Build history of the part. All positions in model axes, mm. Face numbers are marked on the shaded views. Give positions to 0.01 mm unless a question says otherwise; leave off trailing zeros. Loops run counter-clockwise (first coordinate to the right, second up) from the corner with the lowest first, then second, coordinate; pieces in that order, holes last. Notation, with made-up numbers: M -10.75,88 L 19.25,88 A29 cw 19.25,111 Z; hole C 85,-22 d10. An arc over 180 degrees is marked long. Answer in a Markdown table with one row per item. Add a question column.
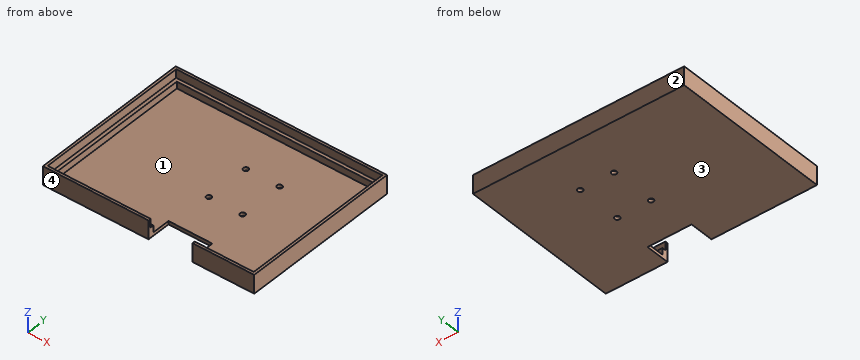
```python
from build123d import *

# Parameters (mm, degrees)
SKETCH1_W           = 125
SKETCH1_H           = 95
SKETCH1_W_2         = 118
SKETCH1_H_2         = 88
BOSS_EXTRUDE1_DEPTH = 4
SKETCH2_W           = 125
SKETCH2_H           = 95
BOSS_EXTRUDE2_DEPTH = 2
SKETCH3_W           = 125
SKETCH3_H           = 95
SKETCH3_W_2         = 122
SKETCH3_H_2         = 92
BOSS_EXTRUDE3_DEPTH = 5
SKETCH5_R           = 1.5
CUT_EXTRUDE1_DEPTH  = 26.5
SKETCH7_W           = 26
SKETCH7_H           = 14.212575567
CUT_EXTRUDE2_DEPTH  = 26.5


with BuildPart() as part:
    # Sketch1 → Boss-Extrude1 (new body)
    with BuildSketch(Plane.XY):
        Rectangle(SKETCH1_W, SKETCH1_H)
        Rectangle(SKETCH1_W_2, SKETCH1_H_2, mode=Mode.SUBTRACT)
    extrude(amount=BOSS_EXTRUDE1_DEPTH)

    # Sketch2 → Boss-Extrude2 (add)
    with BuildSketch(Plane(origin=(0, 0, 0), x_dir=(-1, 0, 0), z_dir=(0, 0, -1))):
        Rectangle(SKETCH2_W, SKETCH2_H)
    extrude(amount=BOSS_EXTRUDE2_DEPTH)

    # Sketch3 → Boss-Extrude3 (add)
    with BuildSketch(Plane.XY.offset(4)):
        Rectangle(SKETCH3_W, SKETCH3_H)
        Rectangle(SKETCH3_W_2, SKETCH3_H_2, mode=Mode.SUBTRACT)
    extrude(amount=BOSS_EXTRUDE3_DEPTH)

    # Sketch5 → Cut-Extrude1 (cut)
    with BuildSketch(Plane(origin=(0, 0, -2), x_dir=(-1, 0, 0), z_dir=(0, 0, -1))):
        with Locations((-23, 18.5)):
            Circle(SKETCH5_R)
        with Locations((-23, -8)):
            Circle(SKETCH5_R)
        with Locations((-3, -8)):
            Circle(SKETCH5_R)
        with Locations((-3, 18.5)):
            Circle(SKETCH5_R)
    extrude(amount=-CUT_EXTRUDE1_DEPTH, mode=Mode.SUBTRACT)

    # Sketch7 → Cut-Extrude2 (cut)
    with BuildSketch(Plane(origin=(0, 0, -2), x_dir=(-1, 0, 0), z_dir=(0, 0, -1))):
        with Locations((-13, -40.393712217)):
            Rectangle(SKETCH7_W, SKETCH7_H)
    extrude(amount=-CUT_EXTRUDE2_DEPTH, mode=Mode.SUBTRACT)


solid = part.part
```
(1) Slice it at D-D, the plane x = 48. Give the cut face in (y, z).
(2) Pin check, flat tips, straight feed: pin 1 (2.5 mm diameter, centred on x = 3, y = 18.5, fed in from -Z); pin 2 (2 mm diameter, centred on x = 16.5, z = -1, fed in from -Y); pin 3 (12 mm diameter, centred on x = -1, y = -3.5, fed in from +Z). Stop position of each tip, or through.
(3) Slice it at B-B, the plane x = 23. Give the cut face in (y, z), then the cut area to 3 significant figures.
(4) Pull direction Y, two halves, no side cores. Call the marked faces 1, 2, 3 and 4: +Y half, -Y half, draft (parallel to the pull), parting line (faces both ways), or undercut.
(5) Slice it at C-C, the plane z = 7. Give the cut face in (x, y).
(6) Wall check: line 1 (Y direction, x = 3, z = -0.75); line 2 (Y direction, x = -3.5, z = 5.5); line 3 (X direction, y = -39, z = 7). Give the ranges that are in metal, low to high.
(7) Slice it at A-A, the plane y = -8. Give the cut face in (x, z).
Solution:
| question | item | result |
|---|---|---|
| 1 | outline | M -47.5,-2 L 47.5,-2 L 47.5,9 L 46,9 L 46,4 L 44,4 L 44,0 L -44,0 L -44,4 L -46,4 L -46,9 L -47.5,9 Z |
| 2 | pin 1 | through |
| 2 | pin 2 | y = -33.29 |
| 2 | pin 3 | z = 0 |
| 3 | outline | M -33.29,-2 L -9.5,-2 L -9.5,0 L -33.29,0 Z; M -6.5,-2 L 17,-2 L 17,0 L -6.5,0 Z; M 20,-2 L 47.5,-2 L 47.5,9 L 46,9 L 46,4 L 44,4 L 44,0 L 20,0 Z |
| 3 | area | 171 mm^2 |
| 4 | face 1 | undercut |
| 4 | face 2 | +Y half |
| 4 | face 3 | draft |
| 4 | face 4 | -Y half |
| 5 | outline | M -62.5,-47.5 L 0,-47.5 L 0,-46 L -61,-46 L -61,46 L 61,46 L 61,-46 L 26,-46 L 26,-47.5 L 62.5,-47.5 L 62.5,47.5 L -62.5,47.5 Z |
| 6 | line 1 | -33.29 to -9.5, -6.5 to 17, 20 to 47.5 |
| 6 | line 2 | -47.5 to -46, 46 to 47.5 |
| 6 | line 3 | -62.5 to -61, 61 to 62.5 |
| 7 | outline | M -62.5,-2 L 1.5,-2 L 1.5,0 L -59,0 L -59,4 L -61,4 L -61,9 L -62.5,9 Z; M 4.5,-2 L 21.5,-2 L 21.5,0 L 4.5,0 Z; M 24.5,-2 L 62.5,-2 L 62.5,9 L 61,9 L 61,4 L 59,4 L 59,0 L 24.5,0 Z |
